Work out the finished part from the listing and answer in its coordinate system (mm). Face numbers are marked on the shaded views. A direction names the side the tool comes from. Round coordinates to 2 decimals unless told otherwise and drop trailing zeros. Order: outer loops, then holes, each group sorted by start corner. A loop starts at its lowest first (then second) coordinate and runs counter-clockwise, first axis right, second up.
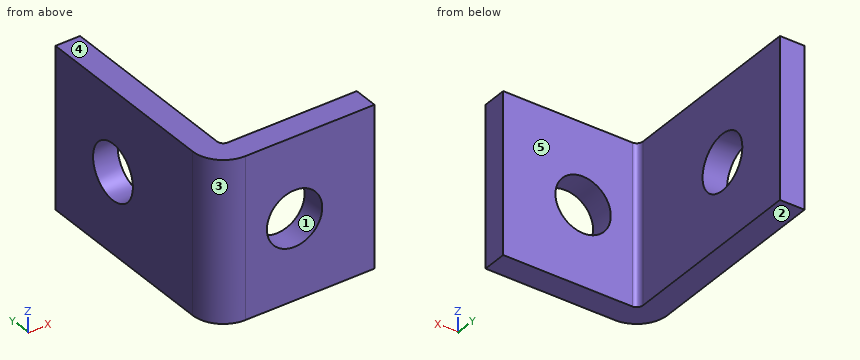
from build123d import *

# Parameters (mm, degrees)
EXTRUDE_THIN1_DEPTH = 20.6375
SKETCH2_R           = 7.14375
CUT_EXTRUDE1_DEPTH  = 69.63069307
SKETCH3_R           = 7.14375
CUT_EXTRUDE2_DEPTH  = 71.084124673


with BuildPart() as part:
    # Sketch1 → Extrude-Thin1 (new, symmetric)
    with BuildSketch(Plane.XY):
        with BuildLine():
            Line((0, 57.15), (0, 7.9375))
            ThreePointArc((0, 7.9375), (2.324839924, 2.324839924), (7.9375, 0))
            Line((7.9375, 0), (41.275, 0))
            Line((41.275, 0), (41.275, 6.35))
            Line((41.275, 6.35), (7.9375, 6.35))
            ThreePointArc((7.9375, 6.35), (6.814967985, 6.814967985), (6.35, 7.9375))
            Line((6.35, 7.9375), (6.35, 57.15))
            Line((6.35, 57.15), (0, 57.15))
        make_face()
    extrude(amount=EXTRUDE_THIN1_DEPTH, both=True)

    # Sketch2 → Cut-Extrude1 (cut, through all)
    with BuildSketch(Plane(origin=(0, 6.35, 0), x_dir=(1, 0, 0), z_dir=(0, 1, 0))):
        with Locations(Location((20.6375, 0, 0), (0, 0, 270))):
            Circle(SKETCH2_R)
    extrude(amount=-CUT_EXTRUDE1_DEPTH, mode=Mode.SUBTRACT)

    # Sketch3 → Cut-Extrude2 (cut, through all)
    with BuildSketch(Plane(origin=(6.35, 0, 0), x_dir=(0, 0, -1), z_dir=(1, 0, 0))):
        with Locations(Location((0, 36.5125, 0), (0, 0, 90))):
            Circle(SKETCH3_R)
    extrude(amount=-CUT_EXTRUDE2_DEPTH, mode=Mode.SUBTRACT)


solid = part.part
Item 1: Find section B-B (x = 4.5). Write down the section's boundary in (y, z), plus the area to 3 significant figures.
Item 2: A tool of negligible diameter and unlimited length cuts with its end or side. For the marked faces 4 and 5, from which of +Z, -Z, +X, -X, +Y, -Y can it reach the whole face along a straight path? Write none if from no direction.
Item 3: Find section D-D (y = 16.5). Write down the section's boundary in (x, z).
Item 4: Find section A-A (z = -4.5). State how many separate pieces and enclosed holes the cut face has, plus the area to 3 significant figures.
Item 5: For a pull along X with two mould halves and no side action, classify the marked faces 1, 2 and 3 as released by +X, released by -X, zero draft, split by the parting line, or undercut.
Item 6: Given pin 1 (16.5 mm diameter, centred on y = 36.51, z = 0, fed in from +X); pin 2 (2 mm diameter, centred on x = 6.5, z = 12.5, fed in from -Y); pin 3 (10 mm diameter, centred on y = 17, z = -6, fed in from -X); pin 4 (11.5 mm diameter, centred on x = 20.64, z = 0, fed in from -Y), each flat-ended and moving along its own axis, determine where each tip first touches the part or whether it passes through.
Item 7: Find the intervals of material crossed by line 1 along X through (y, z) = (53.5, -14); line 2 along X through (y, z) = (3, 0) (3 decimals), in increasing order.
Model answer:
1. outline: (0.78, -20.64) - (57.15, -20.64) - (57.15, 20.64) - (0.78, 20.64) - close; hole circle Ø14.29 at (36.51, 0)
1. area: 2,170 mm2
2. face 4: +Z, +X, -X, +Y, -Y
2. face 5: +Z, -Z, +X, +Y
3. outline: (0, -20.64) - (6.35, -20.64) - (6.35, 20.64) - (0, 20.64) - close
4. separate pieces: 3
4. enclosed holes: 0
4. area: 431 mm2
5. face 1: undercut
5. face 2: zero draft
5. face 3: released by -X
6. pin 1: stops at x = 6.35
6. pin 2: stops at y = 0.01
6. pin 3: stops at x = 0
6. pin 4: passes through
7. line 1: x = 0 to 6.35
7. line 2: x = 1.723 to 13.494, 27.781 to 41.275
